```python
from build123d import *

# Parameters (mm, degrees)
SKETCH_W     = 490
SKETCH_H     = 560
PAD_DEPTH    = 38
FILLET_R     = 4
POCKET_DEPTH = 20
FILLET001_R  = 4
FILLET002_R  = 4
FILLET003_R  = 3


with BuildPart() as part:
    # Sketch → Pad (new body)
    with BuildSketch(Plane.XY):
        with BuildLine():
            Line((0, 0), (45.355339, 45.355339))
            ThreePointArc((80.710678, 60), (61.576507, 56.193977), (45.355339, 45.355339))
            Line((80.710678, 60), (635, 60))
            Line((635, 60), (635, -2500))
            Line((635, -2500), (0, -2500))
            Line((0, -2500), (0, 0))
        make_face()
        with Locations((317.5, -1553.5)):
            Rectangle(SKETCH_W, SKETCH_H, mode=Mode.SUBTRACT)
    extrude(amount=PAD_DEPTH)

    # Fillet
    fillet_edges = [part.edges().sort_by_distance(p)[0] for p in [
        (562.5, -1833.5, 19),
        (562.5, -1273.5, 19),
        (72.5, -1273.5, 19),
        (72.5, -1833.5, 19),
    ]]
    fillet(fillet_edges, radius=FILLET_R)

    # Sketch001 (on Face2 of Fillet) → Pocket (cut)
    with BuildSketch(Plane(origin=(0, 0, 0), x_dir=(1, 0, 0), z_dir=(0, 0, -1))):
        Polygon((105, -60), (105, 10), (80, 35), (80, 70), (140, 70), (140, 35), (115, 10), (115, -60), align=None)
        Polygon((455, -60), (455, 10), (430, 34.999975), (430, 70), (490, 70), (490, 34.999975), (465, 10), (465, -60), align=None)
        Polygon((280, -60), (280, 10), (255, 34.999975), (255, 70), (315, 70), (315, 34.999975), (290, 10), (290, -60), align=None)
    extrude(amount=-POCKET_DEPTH, mode=Mode.SUBTRACT)

    # Fillet001
    fillet001_edges = [part.edges().sort_by_distance(p)[0] for p in [
        (140, -70, 10),
        (140, -35, 10),
        (80, -35, 10),
        (80, -70, 10),
    ]]
    fillet(fillet001_edges, radius=FILLET001_R)

    # Fillet002
    fillet002_edges = [part.edges().sort_by_distance(p)[0] for p in [
        (430, -70, 10),
        (490, -70, 10),
        (490, -34.999975, 10),
        (430, -34.999975, 10),
    ]]
    fillet(fillet002_edges, radius=FILLET002_R)

    # Fillet003
    fillet003_edges = [part.edges().sort_by_distance(p)[0] for p in [
        (315, -70, 10),
        (255, -70, 10),
        (255, -34.999975, 10),
        (315, -34.999975, 10),
    ]]
    fillet(fillet003_edges, radius=FILLET003_R)


solid = part.part
```
Model file for the job. Use its own axes, mm. A direction names the side the tool comes from. Coordinates: 2 decimals unless noted, no trailing zeros. Order: outer loops, then holes, each group sorted by start corner. A loop starts at its lowest first (then second) coordinate and runs counter-clockwise, first axis right, second up. Notation, with made-up numbers: (33.25, 15) - (62.25, 15) arc R16 cw to (62.25, 28) - close; hole circle Ø3 at (72.5, -24.75). An arc over 180 degrees is marked (long way). Return JSON: item names as keys, results as strings. Group by question number.
1) Saw through at A-A, the plane x = 218. Write the cut outline in (y, z), plus the area to 3 significant figures.
2) Tool access for faces 1 (the flat face through (285, -35, 20)), 2 (the flat face through (322, -1202, 38)): list every direction of +Z, -Z, +X, -X, +Y, -Y with a clear straight run to the whole face (end or side of a thin tool).
3) Flat gauge pins, fed straight in: P1, Ø10, axis at y = -2146.5, z = 11.5, coming from the -X side; P2, Ø16, axis at y = 34, z = 11.5, coming from the -X side. Where does each tip first touch, or does it go through?
4) Mould opens along Y. For faces 3 (the flat face through (322, -1202, 0)), 4 (the flat face through (22, 22, 19)), 5 (the flat face through (110, -35, 20)) say: released by +Y, released by -Y, zero draft, split by the parting line, or undercut.
5) Probe line 1 (Y direction, x = 350.5, z = 18); line 2 (X direction, y = -1444, z = 20); line 3 (Y direction, x = 293, z = 19). List the from-to ranges inside material, lowest first. Write a range as from..to.
6) Saw through at B-B, the plane y = -1577. Write the cut outline in (x, z).
7) Saw through at C-C, the plane z = 27. Write the cut outline in (x, y), plus the area to 3 significant figures.
Values found:
{
 "1": {"outline": "(-2500, 0) - (-1833.5, 0) - (-1833.5, 38) - (-2500, 38) - close; (-1273.5, 0) - (60, 0) - (60, 38) - (-1273.5, 38) - close", "area": "76,000 mm²"},
 "2": {"face 1": "-Z", "face 2": "+Z, +X, -X, +Y, -Y"},
 "3": {"P1": "stops at x = 0", "P2": "stops at x = 26"},
 "4": {"face 3": "zero draft", "face 4": "released by +Y", "face 5": "undercut"},
 "5": {"line 1": "y = -2500..-1833.5, -1273.5..60", "line 2": "x = 0..72.5, 562.5..635", "line 3": "y = -2500..-1833.5, -1273.5..-70, -13..60"},
 "6": {"outline": "(0, 0) - (72.5, 0) - (72.5, 38) - (0, 38) - close; (562.5, 0) - (635, 0) - (635, 38) - (562.5, 38) - close"},
 "7": {"outline": "(0, -2500) - (635, -2500) - (635, 60) - (80.71, 60) arc R50 ccw to (45.36, 45.36) - (0, 0) - close; hole (72.5, -1829.5) arc R4 ccw to (76.5, -1833.5) - (558.5, -1833.5) arc R4 ccw to (562.5, -1829.5) - (562.5, -1277.5) arc R4 ccw to (558.5, -1273.5) - (76.5, -1273.5) arc R4 ccw to (72.5, -1277.5) - close", "area": "1,350,000 mm²"}
}
